Study the drawing (mm; zero at the part's minimum x, y, z) and answer. A direction names the side the tool comes from. Give positions to 0.01 mm unless a question says otherwise; leave off trailing zeros. Loops run counter-clockwise (first coordinate to the right, second up) from the corner with the lowest first, then second, coordinate; pieces in that order, holes last. Notation, with made-up numbers: (58.25, -36) - (113.25, -36) arc R22 ccw to (113.25, -12) - close; hole circle Ø4 at (51.5, -24). An arc over 180 degrees is marked (long way). One line per item, written item: value. Start each with the question number.
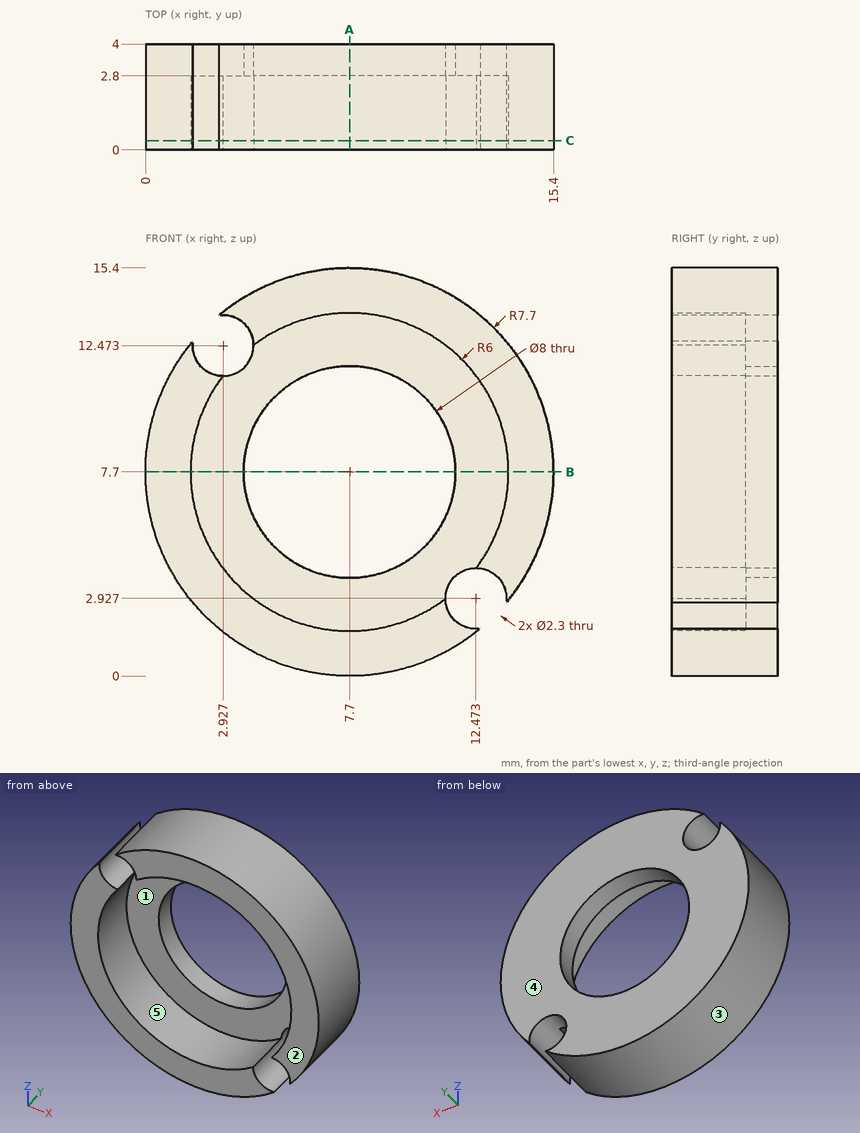
1. A cutting plane is placed at C-C (y = 0.35). Determine the outline of the cut face in (x, z).
2. Determine the mould class of the marked faces 1, 2 and 3 for opening direction X: released by +X, released by -X, zero draft, split by the parting line, or undercut.
3. Flat-ended cylindrical pins translate along their axes: pin 1 (1.5 mm diameter, centred on x = 3, y = 3, fed in from -Z); pin 2 (1.5 mm diameter, centred on x = 12.5, y = 2.5, fed in from +Z); pin 3 (1.5 mm diameter, centred on y = 1.5, z = 11, fed in from +X); pin 4 (5 mm diameter, centred on x = 7.7, z = 7.7, fed in from +Y). Find the tip coordinate at first contact, or state that the pin passes through.
4. For the marked faces 4 and 5, determine the directions among +Z, -Z, +X, -X, +Y, -Y from which every point of the face is accessible in a straight line to the end or side of a thin tool.
5. A cutting plane is placed at A-A (x = 7.7). Determine the outline of the cut face in (y, z), plus the area to 3 significant figures.
6. A cutting plane is placed at B-B (z = 7.7). Determine the outline of the cut face in (x, y).
7. Find the intervals of material crossed by L1, parallel to Z at x = 7.7, y = 3.6; L2, parallel to Z at x = 7.75, y = 1.55; L3, parallel to Y at x = 4, z = 4.75, in increasing order. Write a range as [from, to].
Results below:
1. outline: (1.79, 12.63) arc R7.7 ccw to (12.63, 1.79) arc R1.15 cw to (11.32, 2.92) arc R6 cw to (2.92, 11.32) arc R1.15 cw to start; (2.77, 13.61) arc R1.15 cw to (4.08, 12.48) arc R6 cw to (12.48, 4.08) arc R1.15 cw to (13.61, 2.77) arc R7.7 ccw to start
2. face 1: undercut
2. face 2: zero draft
2. face 3: split by the parting line
3. pin 1: stops at z = 1.09
3. pin 2: stops at z = 14.25
3. pin 3: stops at x = 14.97
3. pin 4: passes through
4. face 4: +Z, -Z, +X, -X, +Y
4. face 5: -Y
5. outline: (0, 0) - (4, 0) - (4, 3.7) - (2.8, 3.7) - (2.8, 1.7) - (0, 1.7) - close; (0, 13.7) - (2.8, 13.7) - (2.8, 11.7) - (4, 11.7) - (4, 15.4) - (0, 15.4) - close
5. area: 18.4 mm^2
6. outline: (0, 0) - (1.7, 0) - (1.7, 2.8) - (3.7, 2.8) - (3.7, 4) - (0, 4) - close; (11.7, 2.8) - (13.7, 2.8) - (13.7, 0) - (15.4, 0) - (15.4, 4) - (11.7, 4) - close
7. L1: z = [0, 3.7], [11.7, 15.4]
7. L2: z = [0, 1.7], [13.7, 15.4]
7. L3: y = [2.8, 4]
